Model file for the job. Use its own axes, mm. Face numbers are marked on the shaded views. A direction names the side the tool comes from. Give positions to 0.01 mm unless a question says otherwise; leave off trailing zeros. Loops run counter-clockwise (first coordinate to the right, second up) from the corner with the lowest first, then second, coordinate; pieces in that order, holes last. Notation, with made-up numbers: M 2.25,-32 L 55.25,-32 A10 cw 55.25,-22 Z; hole C 48,49.25 d8. An arc over 180 degrees is marked long. Answer in a Markdown table with one row per item.
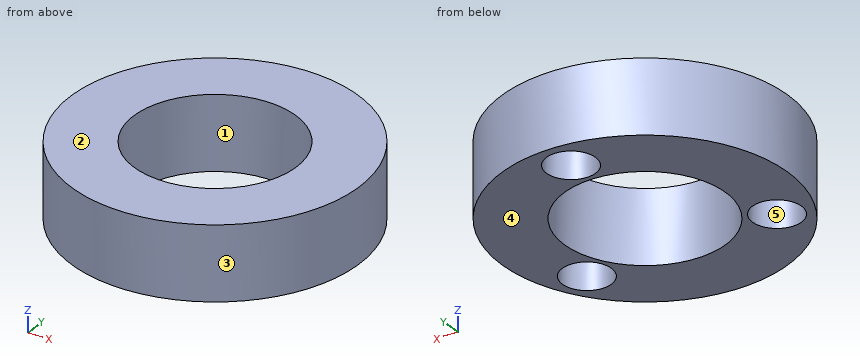
```python
from build123d import *

# Parameters (mm, degrees)
F0_R        = 49.53
F0_R_2      = 8.509
F0_R_3      = 27.94
F1_DEPTH    = 25.4
F1_FACE_R   = 49.53
F1_FACE_R_2 = 27.94
F2_DEPTH    = 10.16


with BuildPart() as f1:
    # F0 (on Top) → F1 (new body)
    with BuildSketch(Plane.XY):
        Circle(F0_R)
        with Locations((-32.9955678842, -19.05)):
            Circle(F0_R_2, mode=Mode.SUBTRACT)
        Circle(F0_R_3, mode=Mode.SUBTRACT)
        with Locations((32.9955678842, -19.05)):
            Circle(F0_R_2, mode=Mode.SUBTRACT)
        with Locations((0.0215684675, 38.0999937206)):
            Circle(F0_R_2, mode=Mode.SUBTRACT)
        with Locations((0.0215684675, 38.0999937206)):
            Circle(F0_R_2)
        with Locations((-32.9955678842, -19.05)):
            Circle(F0_R_2)
        with Locations((32.9955678842, -19.05)):
            Circle(F0_R_2)
    extrude(amount=F1_DEPTH)

    # F1_face (on face) + F0 (on Top) → F2 (cut)
    with BuildSketch(Plane.XY.offset(25.4)):
        Circle(F1_FACE_R)
        Circle(F1_FACE_R_2, mode=Mode.SUBTRACT)
    with BuildSketch(Plane.XY):
        with Locations((0.0215684675, 38.0999937206)):
            Circle(F0_R_2)
        with Locations((-32.9955678842, -19.05)):
            Circle(F0_R_2)
        with Locations((32.9955678842, -19.05)):
            Circle(F0_R_2)
    extrude(amount=F2_DEPTH, mode=Mode.SUBTRACT)


solid = f1.part
```
Q1. Saw through at B-B (x = 6.5). Give the cut face in (y, z), and give its area (3 significant figures).
Reported:
| item | result |
|---|---|
| outline | M -49.1,0 L -27.17,0 L -27.17,25.4 L -49.1,25.4 Z; M 27.17,0 L 32.58,0 L 32.58,10.16 L 43.62,10.16 L 43.62,0 L 49.1,0 L 49.1,25.4 L 27.17,25.4 Z |
| area | 1,000 mm² |
Q2. Probe probe 1 along Y at (x, z) = (-12, 22.75); probe 2 along Y at (x, z) = (2, 16.25). List the from-to ranges inside material, lowest first.
Reported:
| item | result |
|---|---|
| probe 1 | -48.05 to -25.23, 25.23 to 48.05 |
| probe 2 | -49.49 to -27.87, 27.87 to 49.49 |
Q3. Saw through at A-A (y = 0). Give the cut face in (x, z), and give its area (3 significant figures).
Reported:
| item | result |
|---|---|
| outline | M -49.53,0 L -27.94,0 L -27.94,25.4 L -49.53,25.4 Z; M 27.94,0 L 49.53,0 L 49.53,25.4 L 27.94,25.4 Z |
| area | 1,100 mm² |
Q4. Saw through at D-D (z = 15.5). Give the cut face in (x, y).
Reported:
| item | result |
|---|---|
| outline | C 0,0 d99.06; hole C 0,0 d55.88 |
Q5. 3-axis set-ups, long thin cutter, end or side, ignore diameter. For the marked faces 4 and 5: which of +Z, -Z, +X, -X, +Y, -Y reach the whole face in a straight line?
Reported:
| item | result |
|---|---|
| face 4 | -Z, +X, -X, +Y, -Y |
| face 5 | -Z |
Q6. Mould opens along X. For the marked faces 1, 2 and 3 say: released by +X, released by -X, zero draft, split by the parting line, or undercut.
Reported:
| item | result |
|---|---|
| face 1 | undercut |
| face 2 | zero draft |
| face 3 | split by the parting line |
Q7. Drop flat-ended pins along their axis: pin 1 (10 mm diameter, centred on x = 26, z = 11.5, fed in from -Y); pin 2 (1.5 mm diameter, centred on y = -29.5, z = 13.5, fed in from +X); pin 3 (12 mm diameter, centred on x = -20.5, z = 19.5, fed in from -Y); pin 4 (5 mm diameter, centred on x = -13, y = -20.5, fed in from +Z). Give the stop position or say it passes through.
Reported:
| item | result |
|---|---|
| pin 1 | y = -44.86 |
| pin 2 | x = 40.33 |
| pin 3 | y = -47.36 |
| pin 4 | through |
Q8. Saw through at C-C (z = 7.25). Give the cut face in (x, y), and give its area (3 significant figures).
Reported:
| item | result |
|---|---|
| outline | C 0,0 d99.06; hole C -33,-19.05 d17.02; hole C 0,0 d55.88; hole C 0.02,38.1 d17.02; hole C 33,-19.05 d17.02 |
| area | 4,570 mm² |
